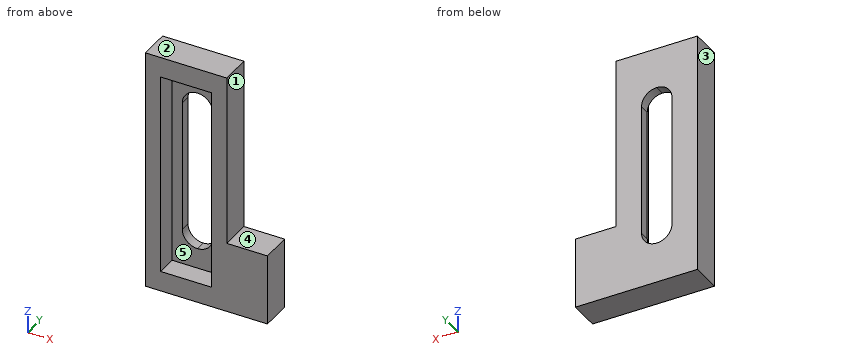
```python
from build123d import *

# Parameters (mm, degrees)
F0_W     = 25
F0_H     = 100
F0_W_2   = 15
F0_H_2   = 80
F1_DEPTH = 15
F2_DEPTH = 10
F3_DEPTH = 15.001
F4_R     = 7.49999


# Not quite as in the source:
# - a fillet or chamfer is up to 0.001 mm smaller than in the source, because OpenCascade refuses the exact size


with BuildPart() as f1:
    # F0 (on Front) → F1 (new body)
    with BuildSketch(Plane.XZ):
        Polygon((20, -25), (20, 60), (-20, 60), (-20, -60), (40, -60), (40, -25), align=None)
        Rectangle(F0_W, F0_H, mode=Mode.SUBTRACT)
        Rectangle(F0_W, F0_H)
        Rectangle(F0_W_2, F0_H_2, mode=Mode.SUBTRACT)
        Rectangle(F0_W_2, F0_H_2)
    extrude(amount=-F1_DEPTH)

    # F0 (on Front) → F2 (cut)
    with BuildSketch(Plane.XZ):
        Rectangle(F0_W, F0_H)
        Rectangle(F0_W_2, F0_H_2, mode=Mode.SUBTRACT)
    extrude(amount=-F2_DEPTH, mode=Mode.SUBTRACT)

    # F0 (on Front) → F3 (cut, through all)
    with BuildSketch(Plane.XZ):
        Rectangle(F0_W_2, F0_H_2)
    extrude(amount=-F3_DEPTH, mode=Mode.SUBTRACT)

    # F4 (radius 7.5 in the source; OpenCascade refuses exactly that, so slightly less here)
    f4_edges = [f1.edges().sort_by_distance(p)[0] for p in [
        (-7.5, 12.5, 40),
        (7.5, 12.5, 40),
        (-7.5, 12.5, -40),
        (7.5, 12.5, -40),
    ]]
    fillet(f4_edges, radius=F4_R)


solid = f1.part
```
Verification items for the finished model (mm, model axes). Face numbers are marked on the shaded views. A direction names the side the tool comes from. Round coordinates to 2 decimals unless told otherwise and drop trailing zeros. Order: outer loops, then holes, each group sorted by start corner. A loop starts at its lowest first (then second) coordinate and runs counter-clockwise, first axis right, second up. Notation, with made-up numbers: (14, 10.5) - (26, 10.5) arc R26 ccw to (26, 43.5) - close; hole circle Ø8 at (18.5, -4). An arc over 180 degrees is marked (long way). Use CSV: the item, a comma, the result in double quotes. Start each with the question number.
1) Section check C-C, the plane x = 9.5. Record the cut outline in (y, z).
2) Thickness scan on L1, parallel to X at y = 10.75, z = 32; L2, parallel to X at y = 4.5, z = -11; L3, parallel to Z at x = -11.5, y = 4.5. Record the ranges inside material, lowest first.
3) Go/stop test with a flat-tipped pin: P1, Ø3, axis at y = 12, z = 44.5, coming from the +X side. Record where the tip stops, or that it passes through.
4) Mould release check, pull along X, two halves, no side actions. Record for the marked faces 3, 4 and 5: +X half, -X half, draft (parallel to the pull), parting line (faces both ways), or undercut.
5) Access from +Z, -Z, +X, -X, +Y, -Y to the whole of each face (thin tool, end or side, straight path). Record for the marked faces 1 and 2.
6) Section check A-A, the plane z = 28. Record the cut outline in (x, y), plus the area to 3 significant figures.
7) Section check D-D, the plane z = -47. Record the cut outline in (x, y).
Answers:
1,outline,"(0, -60) - (15, -60) - (15, 60) - (0, 60) - (0, 50) - (10, 50) - (10, -50) - (0, -50) - close"
2,L1,"x = -20 to -7.5, 7.5 to 20"
2,L2,"x = -20 to -12.5, 12.5 to 20"
2,L3,"z = -60 to -50, 50 to 60"
3,P1,"stops at x = 20"
4,face 3,"-X half"
4,face 4,"draft"
4,face 5,"undercut"
5,face 1,"+Z, +X, +Y, -Y"
5,face 2,"+Z, +X, -X, +Y, -Y"
6,outline,"(-20, 0) - (-12.5, 0) - (-12.5, 10) - (-7.5, 10) - (-7.5, 15) - (-20, 15) - close; (7.5, 10) - (12.5, 10) - (12.5, 0) - (20, 0) - (20, 15) - (7.5, 15) - close"
6,area,"275 mm²"
7,outline,"(-20, 0) - (-12.5, 0) - (-12.5, 10) - (12.5, 10) - (12.5, 0) - (40, 0) - (40, 15) - (-20, 15) - close"
